Input: part model. Units: mm. Frame: model coordinates. Give positions to 0.01 mm unless a question says otherwise; leave off trailing zeros. Write each loop counter-clockwise with the first axis right and the second up, starting at its lowest first coordinate (ties: lowest second). Pieces come first, ordered by that corner, then holes. Notation, with made-up numbers: (-7.75, 35.5) - (36.25, 35.5) arc R26 ccw to (36.25, 50.5) - close; hole circle Ø9 at (-6.75, 44.5). An arc over 180 degrees is marked (long way). Use a Markdown table: item, result. Add a question column.
1. Section query D-D, the plane y = -29.5. Return loops of the section in (x, z).
2. Section query A-A, the plane x = 0. Return loops of the section in (y, z).
3. Section query C-C, the plane y = 5. Return loops of the section in (x, z).
4. Section query B-B, the plane z = 21.05. Count the separate pieces of the cut face and the enclosed holes in it, plus the area to 3 significant figures.
5. Material intervals for probe 1 along X at (y, z) = (-1, 20.45); probe 2 along Y at (x, z) = (-10, 20.35); probe 3 along Y at (x, z) = (-6, 20.6), sorted ascending.
6. Pin query (flat end, axial travel): pin 1 (1.5 mm diameter, centred on x = -29, z = 22, fed in from +Y); pin 2 (3.5 mm diameter, centred on x = 17.76, y = -21, fed in from -Z). Return the tip coordinate at first contact, or that it passes through.
```python
from build123d import *

# Parameters (mm, degrees)
SKETCH_1_R          = 24
SKETCH_1_R_2        = 22
EXTRUDE_1_DEPTH     = 20
SKETCH_2_R          = 42.5
SKETCH_2_R_2        = 22
EXTRUDE_2_DEPTH     = 3
CUT_EXTRUDE_3_DEPTH = 5
SKETCH_12_R         = 24
CUT_EXTRUDE_4_DEPTH = 20
SKETCH_13_R         = 2
CUT_EXTRUDE_7_DEPTH = 30


with BuildPart() as part:
    # 草图1 → 凸台-拉伸1 (new body)
    with BuildSketch(Plane.XY):
        Circle(SKETCH_1_R)
        Circle(SKETCH_1_R_2, mode=Mode.SUBTRACT)
    extrude(amount=EXTRUDE_1_DEPTH)

    # 草图2 → 凸台-拉伸2 (add)
    with BuildSketch(Plane.XY.offset(20)):
        Circle(SKETCH_2_R)
        Circle(SKETCH_2_R_2, mode=Mode.SUBTRACT)
    extrude(amount=EXTRUDE_2_DEPTH)

    # 草图10 → 切除-拉伸3 (cut, symmetric)
    with BuildSketch(Plane.XY.offset(23)):
        with BuildLine():
            ThreePointArc((28.095541398, -13.101166114), (31, 0), (28.095541398, 13.101166114))
            ThreePointArc((28.095541398, 13.101166114), (24.773226276, 14.310389927), (23.564002463, 10.988074805))
            ThreePointArc((23.564002463, 10.988074805), (26, 0), (23.564002463, -10.988074805))
            ThreePointArc((23.564002463, -10.988074805), (24.773226276, -14.310389927), (28.095541398, -13.101166114))
        make_face()
        with BuildLine():
            ThreePointArc((-13.101166114, -28.095541398), (0, -31), (13.101166114, -28.095541398))
            ThreePointArc((13.101166114, -28.095541398), (14.310389927, -24.773226276), (10.988074805, -23.564002463))
            ThreePointArc((10.988074805, -23.564002463), (0, -26), (-10.988074805, -23.564002463))
            ThreePointArc((-10.988074805, -23.564002463), (-14.310389927, -24.773226276), (-13.101166114, -28.095541398))
        make_face()
        with BuildLine():
            ThreePointArc((-28.095541398, 13.101166114), (-31, 0), (-28.095541398, -13.101166114))
            ThreePointArc((-28.095541398, -13.101166114), (-24.773226276, -14.310389927), (-23.564002463, -10.988074805))
            ThreePointArc((-23.564002463, -10.988074805), (-26, 0), (-23.564002463, 10.988074805))
            ThreePointArc((-23.564002463, 10.988074805), (-24.773226276, 14.310389927), (-28.095541398, 13.101166114))
        make_face()
        with BuildLine():
            ThreePointArc((13.101166114, 28.095541398), (0, 31), (-13.101166114, 28.095541398))
            ThreePointArc((-13.101166114, 28.095541398), (-14.310389927, 24.773226276), (-10.988074805, 23.564002463))
            ThreePointArc((-10.988074805, 23.564002463), (0, 26), (10.988074805, 23.564002463))
            ThreePointArc((10.988074805, 23.564002463), (14.310389927, 24.773226276), (13.101166114, 28.095541398))
        make_face()
    extrude(amount=CUT_EXTRUDE_3_DEPTH, both=True, mode=Mode.SUBTRACT)

    # 草图12 → 切除-拉伸4 (cut)
    with BuildSketch(Plane(origin=(0, 0, 0), x_dir=(-1, 0, 0), z_dir=(0, 0, -1))):
        Circle(SKETCH_12_R)
    extrude(amount=-CUT_EXTRUDE_4_DEPTH, mode=Mode.SUBTRACT)

    # 草图13 → 切除-拉伸7 (cut)
    with BuildSketch(Plane.XY):
        with Locations((17.755280905, -21)):
            Circle(SKETCH_13_R)
        with Locations((-17.755280905, -21)):
            Circle(SKETCH_13_R)
        with Locations((17.755280905, 21)):
            Circle(SKETCH_13_R)
        with Locations((-17.755280905, 21)):
            Circle(SKETCH_13_R)
    extrude(amount=CUT_EXTRUDE_7_DEPTH, mode=Mode.SUBTRACT)


solid = part.part
```
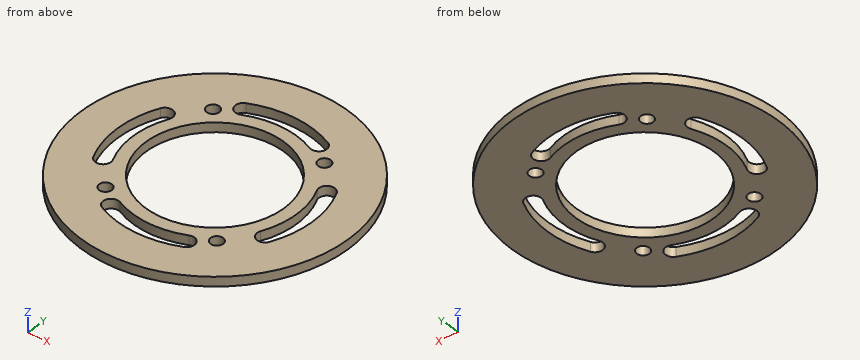
Result sheet:
| question | item | result |
|---|---|---|
| 1 | outline | (-30.59, 20) - (-9.53, 20) - (-9.53, 23) - (-30.59, 23) - close; (9.53, 20) - (30.59, 20) - (30.59, 23) - (9.53, 23) - close |
| 2 | outline | (-42.5, 20) - (-31, 20) - (-31, 23) - (-42.5, 23) - close; (-26, 20) - (-22, 20) - (-22, 23) - (-26, 23) - close; (22, 20) - (26, 20) - (26, 23) - (22, 23) - close; (31, 20) - (42.5, 20) - (42.5, 23) - (31, 23) - close |
| 3 | outline | (-42.2, 20) - (-30.59, 20) - (-30.59, 23) - (-42.2, 23) - close; (-25.51, 20) - (-21.42, 20) - (-21.42, 23) - (-25.51, 23) - close; (21.42, 20) - (25.51, 20) - (25.51, 23) - (21.42, 23) - close; (30.59, 20) - (42.2, 20) - (42.2, 23) - (30.59, 23) - close |
| 4 | separate pieces | 1 |
| 4 | enclosed holes | 9 |
| 4 | area | 3,530 mm² |
| 5 | probe 1 | x = -42.49 to -30.98, -25.98 to -21.98, 21.98 to 25.98, 30.98 to 42.49 |
| 5 | probe 2 | y = -41.31 to -29.34, -24 to -19.6, 19.6 to 24, 29.34 to 41.31 |
| 5 | probe 3 | y = -42.07 to -30.41, -25.3 to -21.17, 21.17 to 25.3, 30.41 to 42.07 |
| 6 | pin 1 | stops at y = 31.75 |
| 6 | pin 2 | passes through |
